from build123d import *

# Parameters (mm, degrees)
F0_W     = 20
F0_H     = 20
F1_DEPTH = 5
F2_W     = 1.5
F2_H     = 1.5
F3_DEPTH = 5
F4_W     = 1.65
F4_H     = 1.65
F5_DEPTH = 5
F6_R     = 0.5


with BuildPart() as f1:
    # F0 (on Top) → F1 (new body)
    with BuildSketch(Plane.XY):
        Rectangle(F0_W, F0_H)
    extrude(amount=F1_DEPTH)

    # F2 (on Top) → F3 (join)
    with BuildSketch(Plane.XY):
        Polygon((-10, -1.5), (-10, 0), (-12.5, 0), (-14, 0), (-14, -1.5), align=None)
        with Locations((-13.25, 0.75)):
            Rectangle(F2_W, F2_H)
    extrude(amount=F3_DEPTH)

    # F4 (on Top) → F5 (cut)
    with BuildSketch(Plane.XY):
        Polygon((10, -1.65), (10, 0.15), (7.5, 0.15), (5.85, 0.15), (5.85, -1.65), align=None)
        with Locations((6.675, 0.975)):
            Rectangle(F4_W, F4_H)
    extrude(amount=F5_DEPTH, mode=Mode.SUBTRACT)

    # F6
    f6_edges = [f1.edges().sort_by_distance(p)[0] for p in [
        (-14, -1.5, 2.5),
        (-14, 1.5, 2.5),
        (-12.5, 1.5, 2.5),
        (-10, 0, 2.5),
        (-12.5, 0, 2.5),
        (-10, -1.5, 2.5),
        (5.85, 1.8, 2.5),
        (7.5, 1.8, 2.5),
        (7.5, 0.15, 2.5),
        (10, 0.15, 2.5),
        (10, -1.65, 2.5),
        (5.85, -1.65, 2.5),
        (10, -10, 2.5),
        (10, 10, 2.5),
        (-10, 10, 2.5),
        (-10, -10, 2.5),
    ]]
    fillet(f6_edges, radius=F6_R)


solid = f1.part
Part model, mm, in its own coordinate system. A direction names the side the tool comes from. Coordinates: 2 decimals unless noted, no trailing zeros. Write each loop counter-clockwise with the first axis right and the second up, starting at its lowest first coordinate (ties: lowest second). Pieces come first, ordered by that corner, then holes. Notation, with made-up numbers: M 83.5,16.5 L 92.5,16.5 A33 cw 92.5,53.5 Z; hole C 76.5,74 d11. An arc over 180 degrees is marked long. Return JSON: item names as keys, results as strings.
1. Pull direction Y, two halves, no side cores. Call faces 1 (the face through (-11, 0, 2)), 2 (the face through (-10, 5, 2)), 3 (the face through (9, 0.15, 2)): pulls with the +Y half, pulls with the -Y half, needs draft (parallel to the pull), parting line crosses it, or undercut.
Determined:
{"face 1": "pulls with the +Y half", "face 2": "needs draft", "face 3": "undercut"}
2. 3-axis set-ups, long thin cutter, end or side, ignore diameter. For faces 4 (the face through (5.85, 0, 2)), 5 (the face through (-12, -1.5, 2)), 6 (the face through (8, -1.65, 2)): which of +Z, -Z, +X, -X, +Y, -Y reach the whole face in a straight line?
Determined:
{"face 4": "+Z, -Z", "face 5": "+Z, -Z, -X, -Y", "face 6": "+Z, -Z, +X"}
3. Saw through at B-B, the plane y = 8. Write the cut outline in (x, z).
Determined:
{"outline": "M -10,0 L 10,0 L 10,5 L -10,5 Z"}
4. Flat gauge pins, fed straight in: pin 1 Ø1.6 at (x, z) = (-11.5, 3.5) entering from +Y; pin 2 Ø3 at (y, z) = (7.5, 4.5) entering from -X. Where does each tip first touch, or does it go through?
Determined:
{"pin 1": "y = 0.1", "pin 2": "x = -10"}
5. Saw through at C-C, the plane x = -11.5. Write the cut outline in (y, z), then the cut area to 3 significant figures.
Determined:
{"outline": "M -1.5,0 L 0,0 L 0,5 L -1.5,5 Z", "area": "7.50 mm²"}
6. Probe L1, parallel to X at y = 0.5, z = 2.8; L2, parallel to Y at x = 8.5, z = 4.1; L3, parallel to Y at x = 7, z = 4.3. List the from-to ranges inside material, lowest first.
Determined:
{"L1": "-14 to -12.5, -10 to 5.85, 7.52 to 9.98", "L2": "-10 to -1.65, 0.15 to 10", "L3": "-10 to -1.65, 1.8 to 10"}
